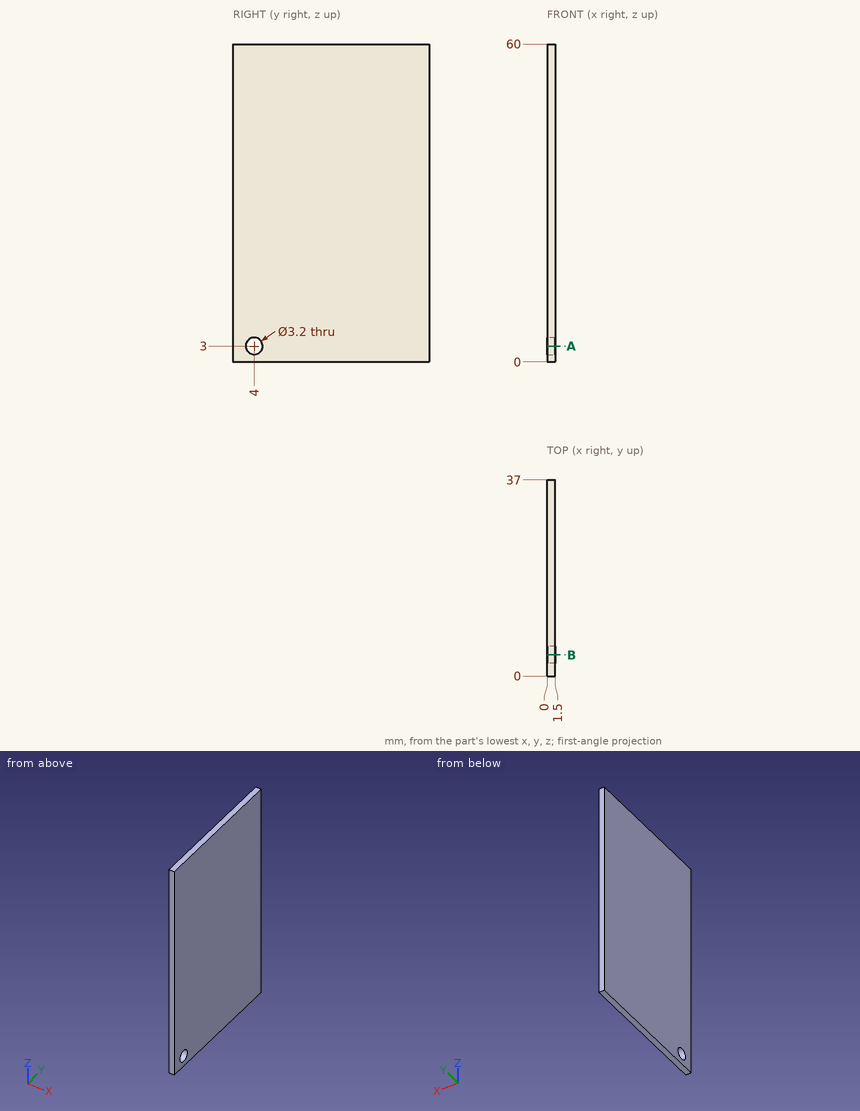
Source: three-view drawing plus pictorial views. Frame: mm from the lowest corner of the part. Round coordinates to 2 decimals unless told otherwise and drop trailing zeros. Loops run counter-clockwise (first coordinate to the right, second up) from the corner with the lowest first, then second, coordinate; pieces in that order, holes last.
Q1. Section B-B, the plane y = 4. Return loops of the section in (x, z).
Q2. First-contact query: P1, Ø2.5, axis at y = 4, z = 3, coming from the +X side. Flat tip, straight axial feed; report the tip coordinate or a pass-through.
Q3. Section A-A, the plane z = 3. Return loops of the section in (x, y), plus the area to 3 significant figures.
Q4. Ray query, line 1 (Y direction, x = 0.4, z = 3). Return the intervals inside material, ascending.
Solutions:
1. outline: (0, 0) - (1.5, 0) - (1.5, 1.4) - (0, 1.4) - close; (0, 4.6) - (1.5, 4.6) - (1.5, 60) - (0, 60) - close
2. P1: passes through
3. outline: (0, 0) - (1.5, 0) - (1.5, 2.4) - (0, 2.4) - close; (0, 5.6) - (1.5, 5.6) - (1.5, 37) - (0, 37) - close
3. area: 50.7 mm2
4. line 1: y = 0 to 2.4, 5.6 to 37
